Can you work these out from the model? Positions are in its coordinate system, mm. Face numbers are marked on the shaded views. A direction names the side the tool comes from. Give positions to 0.01 mm unless a question says otherwise; leave off trailing zeros. Loops run counter-clockwise (first coordinate to the right, second up) from the corner with the lowest first, then second, coordinate; pieces in that order, holes last. Notation, with made-up numbers: (-26.5, 23.25) -> (-1.5, 23.25) arc R25 ccw to (-1.5, 37.25) -> close; hole circle Ø7 at (71.5, 0.5). An arc over 180 degrees is marked (long way). One line per question, with ' | ' between items.
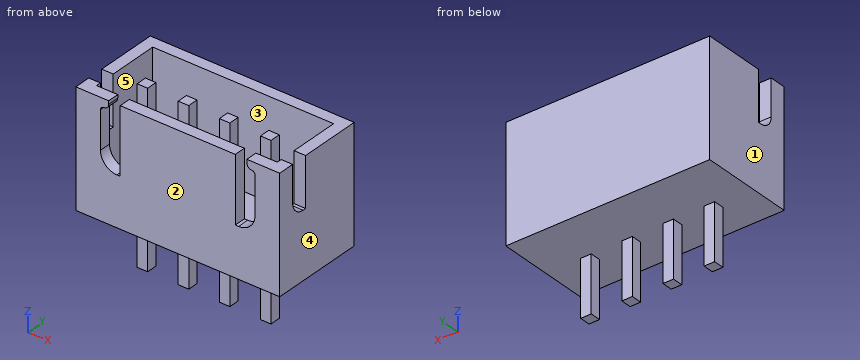
from build123d import *

# Parameters (mm, degrees)
F0_W          = 12.4
F0_H          = 5.75
F0_W_2        = 11
F0_H_2        = 4.35
F0_W_3        = 0.64
F0_H_3        = 0.64
F1_DEPTH      = 1
F2_DEPTH      = 7
F4_DEPTH      = 12.5
F6_DEPTH      = 0.7
F7_DEPTH      = 7
F7_DEPTH_BACK = 3.4


with BuildPart() as f1:
    # F0 (on Top) → F1 (new body)
    with BuildSketch(Plane.XY):
        with Locations((6.2, 2.875)):
            Rectangle(F0_W, F0_H)
        with Locations((6.2, 2.875)):
            Rectangle(F0_W_2, F0_H_2, mode=Mode.SUBTRACT)
        with Locations((6.2, 2.875)):
            Rectangle(F0_W_2, F0_H_2)
        with Locations((2.45, 2.35)):
            Rectangle(F0_W_3, F0_H_3, mode=Mode.SUBTRACT)
        with Locations((4.95, 2.35)):
            Rectangle(F0_W_3, F0_H_3, mode=Mode.SUBTRACT)
        with Locations((7.45, 2.35)):
            Rectangle(F0_W_3, F0_H_3, mode=Mode.SUBTRACT)
        with Locations((9.95, 2.35)):
            Rectangle(F0_W_3, F0_H_3, mode=Mode.SUBTRACT)
    extrude(amount=F1_DEPTH)

    # F0 (on Top) → F2 (join)
    with BuildSketch(Plane.XY):
        with Locations((6.2, 2.875)):
            Rectangle(F0_W, F0_H)
        with Locations((6.2, 2.875)):
            Rectangle(F0_W_2, F0_H_2, mode=Mode.SUBTRACT)
    extrude(amount=F2_DEPTH)

    # F3 (on face) → F4 (cut)
    with BuildSketch(Plane.YZ.offset(12.4)):
        with BuildLine():
            Line((2, 7), (1, 7))
            Line((1, 7), (1, 4.8))
            ThreePointArc((1, 4.8), (1.2343145751, 4.2343145751), (1.8, 4))
            Line((1.8, 4), (2, 4))
            Line((2, 4), (2, 7))
        make_face()
    extrude(amount=-F4_DEPTH, mode=Mode.SUBTRACT)

    # F5 (on face) → F6 (cut)
    with BuildSketch(Plane.XZ):
        with BuildLine():
            Line((2.7, 3), (2.7, 7))
            Line((2.7, 7), (2, 7))
            Line((2, 7), (2, 6.8))
            ThreePointArc((2, 6.8), (1.9121320344, 6.5878679656), (1.7, 6.5))
            ThreePointArc((1.7, 6.5), (1.5585786438, 6.4414213562), (1.5, 6.3))
            Line((1.5, 6.3), (1.5, 4))
            ThreePointArc((1.5, 4), (1.7928932188, 3.2928932188), (2.5, 3))
            Line((2.5, 3), (2.7, 3))
        make_face()
        with BuildLine():
            Line((10.4, 7), (9.7, 7))
            Line((9.7, 7), (9.7, 3))
            Line((9.7, 3), (9.9, 3))
            ThreePointArc((9.9, 3), (10.6071067812, 3.2928932188), (10.9, 4))
            Line((10.9, 4), (10.9, 6.3))
            ThreePointArc((10.9, 6.3), (10.8414213562, 6.4414213562), (10.7, 6.5))
            ThreePointArc((10.7, 6.5), (10.4878679656, 6.5878679656), (10.4, 6.8))
            Line((10.4, 6.8), (10.4, 7))
        make_face()
    extrude(amount=-F6_DEPTH, mode=Mode.SUBTRACT)

    # F0 (on Top) → F7 (join, two sides)
    with BuildSketch(Plane.XY) as f7_sk:
        with Locations((2.45, 2.35)):
            Rectangle(F0_W_3, F0_H_3)
        with Locations((4.95, 2.35)):
            Rectangle(F0_W_3, F0_H_3)
        with Locations((7.45, 2.35)):
            Rectangle(F0_W_3, F0_H_3)
        with Locations((9.95, 2.35)):
            Rectangle(F0_W_3, F0_H_3)
    extrude(amount=F7_DEPTH)
    extrude(f7_sk.sketch, amount=-F7_DEPTH_BACK)


solid = f1.part
Q1. If we section it at C-C (z = -2): Write out the boundary of the cut face in (x, y), plus the area to 3 significant figures.
Entries:
outline: (2.13, 2.03) -> (2.77, 2.03) -> (2.77, 2.67) -> (2.13, 2.67) -> close; (4.63, 2.03) -> (5.27, 2.03) -> (5.27, 2.67) -> (4.63, 2.67) -> close; (7.13, 2.03) -> (7.77, 2.03) -> (7.77, 2.67) -> (7.13, 2.67) -> close; (9.63, 2.03) -> (10.27, 2.03) -> (10.27, 2.67) -> (9.63, 2.67) -> close | area: 1.64 mm²
Q2. For pin 1 Ø1.7 at (x, y) = (4, 3.5) entering from -Z; pin 2 Ø0.5 at (y, z) = (2, -1) entering from -X; pin 3 Ø0.7 at (y, z) = (2.5, -2) entering from +X, each with a flat end and sliding along its axis, tell me the tip position at first contact or that it passes through.
Entries:
pin 1: z = 0 | pin 2: x = 2.13 | pin 3: x = 10.27
Q3. If we section it at D-D (x = 3.25): Write out the boundary of the cut face in (y, z).
Entries:
outline: (0, 0) -> (5.75, 0) -> (5.75, 7) -> (5.05, 7) -> (5.05, 1) -> (0.7, 1) -> (0.7, 7) -> (0, 7) -> close
Q4. If I drill on probe 1 along Y at (x, z) = (2.5, 1.25); probe 2 along X at (y, z) = (2.45, 4); probe 3 along X at (y, z) = (3, 4), over which ranges is the centre line in solid material (lowest first)? Write a range as from..to.
Entries:
probe 1: 0..0.7, 2.03..2.67, 5.05..5.75 | probe 2: 0..0.7, 2.13..2.77, 4.63..5.27, 7.13..7.77, 9.63..10.27, 11.7..12.4 | probe 3: 0..0.7, 11.7..12.4
Q5. If we section it at A-A (z = 2.5): Write out the boundary of the cut face in (x, y).
Entries:
outline: (0, 0) -> (12.4, 0) -> (12.4, 5.75) -> (0, 5.75) -> close; (2.13, 2.03) -> (2.77, 2.03) -> (2.77, 2.67) -> (2.13, 2.67) -> close; (4.63, 2.03) -> (5.27, 2.03) -> (5.27, 2.67) -> (4.63, 2.67) -> close; (7.13, 2.03) -> (7.77, 2.03) -> (7.77, 2.67) -> (7.13, 2.67) -> close; (9.63, 2.03) -> (10.27, 2.03) -> (10.27, 2.67) -> (9.63, 2.67) -> close; hole (0.7, 0.7) -> (11.7, 0.7) -> (11.7, 5.05) -> (0.7, 5.05) -> close
Q6. If we section it at B-B (y = 0.4): Write out the boundary of the cut face in (x, z).
Entries:
outline: (0, 0) -> (12.4, 0) -> (12.4, 7) -> (10.4, 7) -> (10.4, 6.8) arc R0.3 ccw to (10.7, 6.5) arc R0.2 cw to (10.9, 6.3) -> (10.9, 4) arc R1 cw to (9.9, 3) -> (9.7, 3) -> (9.7, 7) -> (2.7, 7) -> (2.7, 3) -> (2.5, 3) arc R1 cw to (1.5, 4) -> (1.5, 6.3) arc R0.2 cw to (1.7, 6.5) arc R0.3 ccw to (2, 6.8) -> (2, 7) -> (0, 7) -> close
Q7. On a 3-axis mill with a long thin cutter (end or side, diameter ignored), from which of +Z, -Z, +X, -X, +Y, -Y can I reach the whole of each face in a straight line? I mean the marked faces 4 and 5. Say none if no direction works.
Entries:
face 4: +Z, -Z, +X, +Y, -Y | face 5: +Z
Q8. If we mould it in two halves opening along X, with no side actions, what happens to the marked faces 1, 2 and 3? For each: pulls with the +X half, pulls with the -X half, needs draft (parallel to the pull), parting line crosses it, or undercut.
Entries:
face 1: pulls with the -X half | face 2: needs draft | face 3: undercut
